Could you check a few things on this model? Use its own coordinates, in mm. A direction names the side the tool comes from. Round coordinates to 2 decimals unless told otherwise and drop trailing zeros. Order: outer loops, then holes, each group sorted by start corner. A loop starts at its lowest first (then second) coordinate and runs counter-clockwise, first axis right, second up. Notation, with made-up numbers: (-28.75, -33.75) - (12.25, -33.75) arc R12 ccw to (12.25, -23.75) - close; hole circle Ø1 at (78.25, -24). An arc over 180 degrees is marked (long way). Use one line per item in the form item = value.
from build123d import *

# Parameters (mm, degrees)
BOSS_EXTRUDE1_DEPTH = 6
SKETCH8_R           = 10.05
CUT_EXTRUDE4_DEPTH  = 4.5
SKETCH9_R           = 7.975
CUT_EXTRUDE5_DEPTH  = 5.1
SKETCH10_R          = 2.55
CUT_EXTRUDE6_DEPTH  = 1.9
SKETCH11_R          = 1.55
CUT_EXTRUDE7_DEPTH  = 2.5
CHAMFER1_SIZE       = 0.5


with BuildPart() as part:
    # Sketch4 → Boss-Extrude1 (new body)
    with BuildSketch(Plane.XY):
        with BuildLine():
            Line((-25, 15), (25, 15))
            ThreePointArc((25, 15), (40, 0), (25, -15))
            Line((25, -15), (-25, -15))
            ThreePointArc((-25, -15), (-40, 0), (-25, 15))
        make_face()
    extrude(amount=BOSS_EXTRUDE1_DEPTH)

    # Sketch8 → Cut-Extrude4 (cut)
    with BuildSketch(Plane.XY.offset(6)):
        with Locations((-25, 0)):
            Circle(SKETCH8_R)
    extrude(amount=-CUT_EXTRUDE4_DEPTH, mode=Mode.SUBTRACT)

    # Sketch9 → Cut-Extrude5 (cut)
    with BuildSketch(Plane(origin=(0, 0, 0), x_dir=(-1, 0, 0), z_dir=(0, 0, -1))):
        with Locations((-25, 0)):
            Circle(SKETCH9_R)
    extrude(amount=-CUT_EXTRUDE5_DEPTH, mode=Mode.SUBTRACT)

    # Sketch10 → Cut-Extrude6 (cut, through all)
    with BuildSketch(Plane(origin=(0, 0, 5.1), x_dir=(-1, 0, 0), z_dir=(0, 0, -1))):
        with Locations((-25, 0)):
            Circle(SKETCH10_R)
    extrude(amount=-CUT_EXTRUDE6_DEPTH, mode=Mode.SUBTRACT)

    # Sketch11 → Cut-Extrude7 (cut, through all)
    with BuildSketch(Plane.XY.offset(1.5)):
        with Locations((-25, 0)):
            Circle(SKETCH11_R)
        with Locations((-18, 0)):
            Circle(SKETCH11_R)
        with Locations((-32, 0)):
            Circle(SKETCH11_R)
        with Locations((-25, 7)):
            Circle(SKETCH11_R)
        with Locations((-25, -7)):
            Circle(SKETCH11_R)
    extrude(amount=-CUT_EXTRUDE7_DEPTH, mode=Mode.SUBTRACT)

    # Chamfer1
    chamfer1_edges = [part.edges().sort_by_distance(p)[0] for p in [
        (-35.05, 0, 6),
        (32.975, 0, 0),
    ]]
    chamfer(chamfer1_edges, length=CHAMFER1_SIZE)


solid = part.part
Item 1: Imagine slicing it at A-A on y = 0. State how many separate pieces and enclosed holes the cut face has, plus the area to 3 significant figures.
Found:
separate_pieces = 5
enclosed_holes = 0
area = 289 mm2
Item 2: Imagine slicing it at C-C on x = 34.5. Please give me the cut outline in (y, z), plus the area to 3 significant figures.
Found:
outline = (-11.61, 0) - (11.61, 0) - (11.61, 6) - (-11.61, 6) - close
area = 139 mm2
Item 3: I need wall thicknesses on L1, parallel to Y at x = -25, z = 0.4; L2, parallel to X at y = 0.5, z = 4.3; L3, parallel to X at y = 6, z = 4.5. Which ranges of each line are inside material? Lowest first, please.
Found:
L1 = -15 to -8.55, -5.45 to -1.55, 1.55 to 5.45, 8.55 to 15
L2 = -39.99 to -35.04, -14.96 to 17.04, 32.96 to 39.99
L3 = -38.75 to -33.06, -16.94 to 19.75, 30.25 to 38.75
Item 4: For faces 4 (the face through (27, 2, 5.1)), 5 (the face through (27.548, 0.112, 5.544)), 6 (the face through (-25, -2, 1.5)), which set-ups out of +Z, -Z, +X, -X, +Y, -Y let a thin tool reach every point of the face, with its end or its side?
Found:
face_4 = -Z
face_5 = +Z, -Z
face_6 = +Z
Item 5: If we mould it in two halves opening along Y, with no side actions, what happens to faces 1 (the face through (1, 0, 0)), 2 (the face through (40, 0, 3)), 3 (the face through (-35.04, 0.44, 3.53))? For each: released by +Y, released by -Y, zero draft, split by the parting line, or undercut.
Found:
face_1 = zero draft
face_2 = split by the parting line
face_3 = undercut
Item 6: Imagine slicing it at B-B on z = 3.1. Please give me the cut outline in (x, y) (3 decimals), plus the area to 3 significant figures.
Found:
outline = (-25, -15) - (25, -15) arc R15 ccw to (25, 15) - (-25, 15) arc R15 ccw to start; hole circle Ø20.1 at (-25, 0); hole circle Ø15.95 at (25, 0)
area = 1,690 mm2
Item 7: Will these pins go through, and if not, where does the flat tip stop? P1, Ø3, axis at x = -18, y = 0, coming from the +Z side; P2, Ø4, axis at x = -25, y = 0, coming from the -Z side; P3, Ø4, axis at x = 28, y = 5.5, coming from the -Z side; P4, Ø5, axis at x = -25, y = 7, coming from the +Z side.
Found:
P1 = through
P2 = 0
P3 = 0.21
P4 = 1.5
